from build123d import *

# Parameters (mm, degrees)
F1_DEPTH = 76.2
F2_DEPTH = 25.4
F3_R     = 12.201191
F4_DEPTH = 50.8


with BuildPart() as f1:
    # F0 (on Front) → F1 (new body)
    with BuildSketch(Plane.XZ):
        Polygon((69.451064, -56.958791), (0, 28.405037), (-57.55366, 28.405037), (-57.55366, -56.958791), align=None)
    extrude(amount=F1_DEPTH)

    # F0 (on Front) → F2 (join)
    with BuildSketch(Plane.XZ):
        Polygon((69.451064, -56.958791), (0, 28.405037), (-57.55366, 28.405037), (-57.55366, -56.958791), align=None)
        Polygon((-57.55366, 28.405037), (0, 28.405037), (69.451064, -56.958791), (81.550552, -56.958791), (0, 43.276783), (-57.55366, 43.276783), align=None)
    extrude(amount=-F2_DEPTH)

    # F3 (on face) → F4 (cut)
    with BuildSketch(Plane(origin=(13.905559, 0, 11.313409), x_dir=(0, 1, 0), z_dir=(0.7757, 0, 0.631101))):
        with Locations((-38.1, -29.861083)):
            Circle(F3_R)
    extrude(amount=-F4_DEPTH, mode=Mode.SUBTRACT)


solid = f1.part
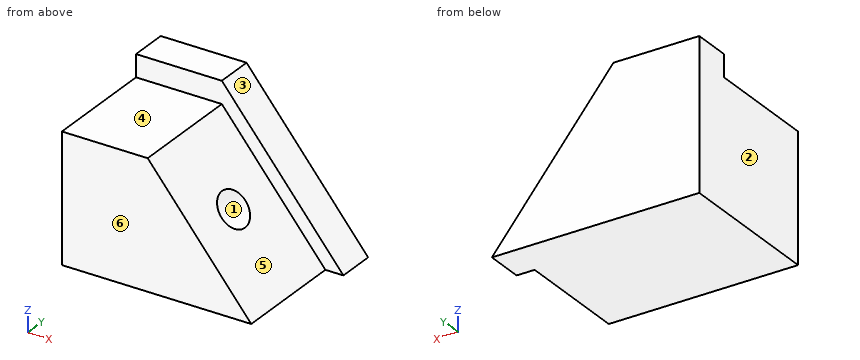
Can you work these out from the model? Positions are in its coordinate system, mm. Face numbers are marked on the shaded views. A direction names the side the tool comes from. Coordinates: 2 decimals unless noted, no trailing zeros. Loops run counter-clockwise (first coordinate to the right, second up) from the corner with the lowest first, then second, coordinate; pieces in that order, holes last. Notation, with made-up numbers: (81, 41.25) - (115, 41.25) arc R15 cw to (115, 68.25) - close; hole circle Ø2 at (-21, 46.5). An arc over 180 degrees is marked (long way). Put each result on its own line as item: value. Start each with the question number.
Item 1: Suppose I cut it at C-C (z = 6.5). Please give me the cut outline in (x, y).
Item 2: If we mould it in two halves opening along Z, with no side actions, what happens to the marked faces 1, 2 and 3? For each: +Z half, -Z half, draft (parallel to the pull), parting line (faces both ways), or undercut.
Item 3: Suppose I cut it at B-B (x = 44). Please give me the cut outline in (y, z).
Item 4: For pin 1 (1.5 mm diameter, centred on y = -17, z = -2, fed in from +X); pin 2 (5 mm diameter, centred on y = -39.5, z = 26, fed in from +X); pin 3 (2 mm diameter, centred on y = -27.5, z = -46, fed in from +X), each with a flat end and sliding along its axis, tell me the tip position at first contact or that it passes through.
Item 5: Suppose I cut it at A-A (y = -29.5). Please give me the cut outline in (x, z).
Item 6: Suppose I cut it at D-D (y = -58). Please give me the cut outline in (x, z).
Item 7: Which directions (+Z, -Z, +X, -X, +Y, -Y) give clear straight access to the entire face, cutting with the end or side of a thin tool? Please do the marked faces 4, 5 and 6.
Item 8: If I drill on line 1 along Y through (x, z) = (12, -29); line 2 along Z through (x, y) = (-13, -24.5); line 3 along Y through (x, z) = (25, -30), over which ranges is the centre line in solid material (lowest first)?
Here are the results:
1. outline: (-57.55, -76.2) - (17.82, -76.2) - (17.82, 0) - (29.92, 0) - (29.92, 25.4) - (-57.55, 25.4) - close
2. face 1: undercut
2. face 2: draft
2. face 3: +Z half
3. outline: (-76.2, -56.96) - (25.4, -56.96) - (25.4, -10.8) - (0, -10.8) - (0, -25.68) - (-76.2, -25.68) - close
4. pin 1: x = 25.35
4. pin 2: x = 3.99
4. pin 3: x = 61.35
5. outline: (-57.55, -56.96) - (69.45, -56.96) - (38.21, -18.56) - (-1.19, -50.62) - (-12.12, -37.2) - (27.29, -5.14) - (0, 28.41) - (-57.55, 28.41) - close
6. outline: (-57.55, -56.96) - (69.45, -56.96) - (0, 28.41) - (-57.55, 28.41) - close
7. face 4: +Z, +X, -X, -Y
7. face 5: +Z, +X, -Y
7. face 6: +Z, -Z, +X, -X, -Y
8. line 1: -76.2 to -50.3, -25.9 to 25.4
8. line 2: -56.96 to 28.41
8. line 3: -76.2 to -46.13, -30.07 to 25.4
